from build123d import *

# Parameters (mm, degrees)
F0_W     = 3
F0_H     = 29
F1_DEPTH = 2.5
F6_R     = 1.24999
F7_W     = 3
F7_H     = 2
F8_DEPTH = 2


# Not quite as in the source:
# - a fillet or chamfer is up to 0.001 mm smaller than in the source, because OpenCascade refuses the exact size


with BuildPart() as f1:
    # F0 (on Top) → F1 (new body)
    with BuildSketch(Plane.XY):
        with Locations((-28.6103483079, 8.1154592335)):
            Rectangle(F0_W, F0_H)
    extrude(amount=F1_DEPTH)

    # F2 (on face) → F3 (revolve, cut)
    with BuildSketch(Plane.YZ.offset(-27.1103483079)):
        with BuildLine():
            Line((-3.3845407665, 0.25), (-3.3845407665, 2.25))
            ThreePointArc((-3.3845407665, 2.25), (-4.3845407665, 1.25), (-3.3845407665, 0.25))
        make_face()
    revolve(axis=Axis((-27.1103483079, -3.3845407665, 1.25), (0, 0, -1)), mode=Mode.SUBTRACT)

    # F4 (on face) → F5 (revolve, cut)
    with BuildSketch(Plane(origin=(-30.1103483079, 0, 0), x_dir=(0, -1, 0), z_dir=(-1, 0, 0))):
        with BuildLine():
            Line((2.3845407665, 1.25), (4.3845407665, 1.25))
            ThreePointArc((4.3845407665, 1.25), (3.3845407665, 2.25), (2.3845407665, 1.25))
        make_face()
    revolve(axis=Axis((-30.1103483079, -3.3845407665, 1.25), (0, -1, 0)), mode=Mode.SUBTRACT)

    # F6 (radius 1.25 in the source; OpenCascade refuses exactly that, so slightly less here)
    f6_edges = [f1.edges().sort_by_distance(p)[0] for p in [
        (-28.610348, -6.384541, 2.5),
        (-28.610348, -6.384541, 0),
    ]]
    fillet(f6_edges, radius=F6_R)

    # F7 (on face) → F8 (cut)
    with BuildSketch(Plane(origin=(0, 0, 0), x_dir=(1, 0, 0), z_dir=(0, 0, -1))):
        with Locations((-28.6103483079, -20.6154592335)):
            Rectangle(F7_W, F7_H)
    extrude(amount=-F8_DEPTH, mode=Mode.SUBTRACT)


solid = f1.part
The model under review builds one solid part; all positions refer to its coordinate system, in mm. A direction names the side the tool comes from. Coordinates: 2 decimals unless noted, no trailing zeros. Loops run counter-clockwise (first coordinate to the right, second up) from the corner with the lowest first, then second, coordinate; pieces in that order, holes last.
(1) Draft analysis for pull direction Y (two halves, no side actions). For faces 3 (the flat face through (-29, 9, 2.5)), 4 (the cylindrical face through (-28.59, -6.03, 0.38)), 5 (the flat face through (-29, 21, 2)), state which applies: +Y half, -Y half, draft (parallel to the pull), parting line (faces both ways), or undercut.
Determined:
face 3: draft
face 4: -Y half
face 5: undercut
(2) Consider section C-C, the plane y = -3. Give the boundary of the cut face in (x, z).
Determined:
outline: (-30.11, 0) - (-27.11, 0) - (-27.11, 0.33) arc R0.92 cw to (-27.11, 2.17) - (-27.11, 2.5) - (-30.11, 2.5) - (-30.11, 2.17) arc R0.92 cw to (-30.11, 0.33) - close
(3) Wall thickness on L1, parallel to Y at x = -29.3, z = 1.65; L2, parallel to Y at x = -27.9, z = 0.9; L3, parallel to Z at x = -27.85, y = -3.75: over which ranges is each line inside the solid? List them lowest first.
Determined:
L1: y = -6.32 to -3.81, -2.96 to 19.62, 21.62 to 22.62
L2: y = -6.33 to -3.89, -2.88 to 19.62, 21.62 to 22.62
L3: z = 0 to 0.68, 1.82 to 2.5
(4) Tool access review of faces 1 (the cylindrical face through (-28.59, -6.03, 2.12)), 2 (the flat face through (-29, 19.615, 1)): name each direction out of +Z, -Z, +X, -X, +Y, -Y from which nothing blocks a thin tool from reaching the whole face with its end or side.
Determined:
face 1: +Z, +X, -X, -Y
face 2: -Z, +X, -X
(5) Consider section B-B, the plane z = 1.65. Give the boundary of the cut face in (x, y).
Determined:
outline: (-30.11, -6.32) - (-27.11, -6.32) - (-27.11, -4.3) arc R0.92 cw to (-27.11, -2.47) - (-27.11, 19.62) - (-30.11, 19.62) - (-30.11, -2.47) arc R0.92 cw to (-30.11, -4.3) - close; (-30.11, 21.62) - (-27.11, 21.62) - (-27.11, 22.62) - (-30.11, 22.62) - close
